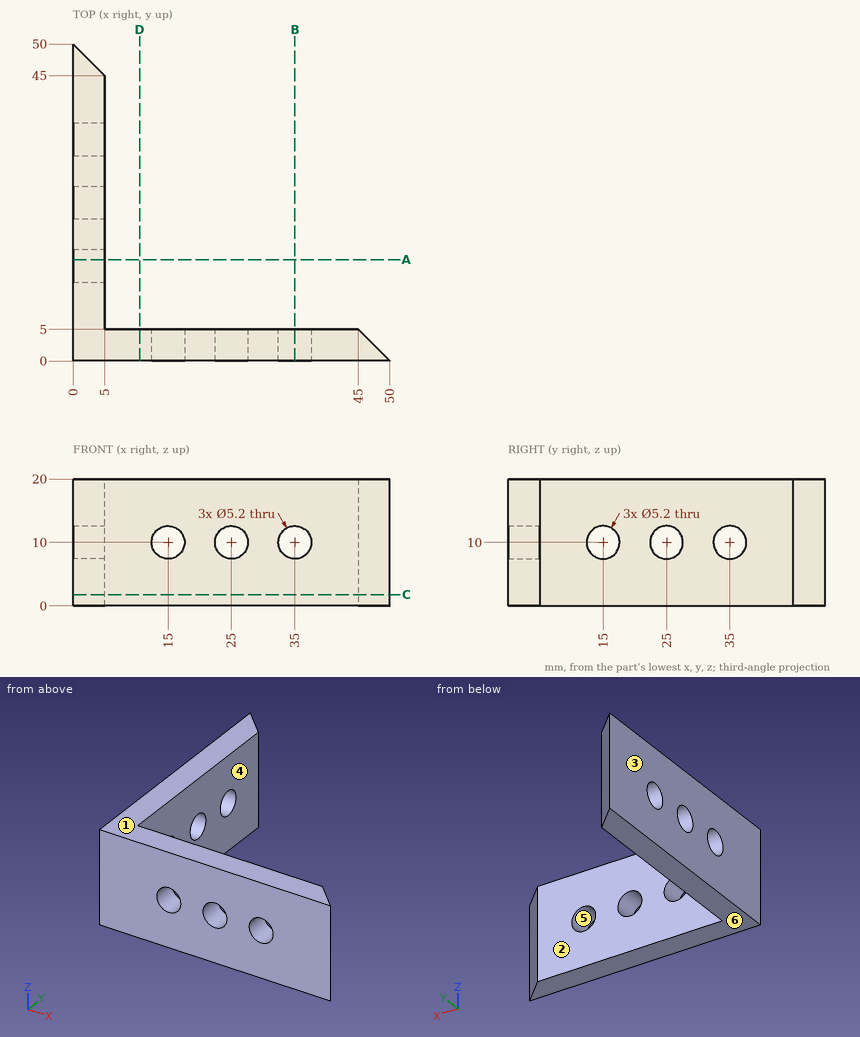
The drawing under review shows one solid part. Ordinate dimensions are in mm from its lowest x, y, z. A direction names the side the tool comes from. Coordinates: 2 decimals unless noted, no trailing zeros. Write each loop counter-clockwise with the first axis right and the second up, starting at its lowest first coordinate (ties: lowest second). Pieces come first, ordered by that corner, then holes. Notation, with made-up numbers: (43, -34.5) -> (98, -34.5) arc R22 cw to (98, -8.5) -> close; hole circle Ø6 at (-35, 70). An arc over 180 degrees is marked (long way). Write each question's results on one line, items separated by ' | '. Start each with the question number.
1) Wall thickness on L1, parallel to Y at x = 1.1, z = 10; L2, parallel to Z at x = 15, y = 3.95; L3, parallel to Y at x = 1.3, z = 10: over which ranges is each line inside the solid? List them lowest first. Write a range as [from, to].
2) Consider section D-D (x = 10.5). Write out the cut boundary in (y, z), plus the area to 3 significant figures.
3) Insertion check: pin 1 (3 mm diameter, centred on x = 30.5, z = 8.5, fed in from +Y); pin 2 (4 mm diameter, centred on x = 25, z = 10, fed in from +Y); pin 3 (3 mm diameter, centred on y = 34.5, z = 12.5, fed in from +X). Each pin has a flat end and moves straight along its axis. Give the tip position at first contact, or say it passes through.
4) The part is to be moulded in two halves that separate along X. For the marked faces 3, 4, 5 and 6, say which applies: +X half, -X half, draft (parallel to the pull), parting line (faces both ways), or undercut.
5) Consider section C-C (z = 1.75). Write out the cut boundary in (x, y).
6) For the marked faces 1 and 2, list the 3-axis set-ups (+Z, -Z, +X, -X, +Y, -Y) from which the entire face can be reached by the end or side of a thin tool; tool diameter is ignored.
7) Consider section B-B (x = 35). Write out the cut boundary in (y, z).
8) Consider section A-A (y = 16). Write out the cut boundary in (x, z), plus the area to 3 significant figures.
Geometry says:
1) L1: [0, 12.4], [17.6, 22.4], [27.6, 32.4], [37.6, 48.9] | L2: [0, 7.4], [12.6, 20] | L3: [0, 12.4], [17.6, 22.4], [27.6, 32.4], [37.6, 48.7]
2) outline: (0, 0) -> (5, 0) -> (5, 20) -> (0, 20) -> close | area: 100 mm^2
3) pin 1: y = 5 | pin 2: through | pin 3: x = 5
4) face 3: -X half | face 4: +X half | face 5: undercut | face 6: draft
5) outline: (0, 0) -> (50, 0) -> (45, 5) -> (5, 5) -> (5, 45) -> (0, 50) -> close
6) face 1: +Z, +X, -X, +Y, -Y | face 2: +Z, -Z, +X, +Y
7) outline: (0, 0) -> (5, 0) -> (5, 7.4) -> (0, 7.4) -> close; (0, 12.6) -> (5, 12.6) -> (5, 20) -> (0, 20) -> close
8) outline: (0, 0) -> (5, 0) -> (5, 7.6) -> (0, 7.6) -> close; (0, 12.4) -> (5, 12.4) -> (5, 20) -> (0, 20) -> close | area: 76.0 mm^2
